from build123d import *
from build123d.topology import SkipClean

# Parameters (mm, degrees)
SKETCH1_R               = 10.5
SKETCH1_R_2             = 4
BOSS_EXTRUDE1_DEPTH     = 10
SKETCH1_3_R             = 4
BOSS_EXTRUDE2_DEPTH     = 17
CUT_EXTRUDE3_DEPTH      = 38.101212918
CUT_EXTRUDE3_DEPTH_BACK = 38.101212918
SKETCH4_R               = 5
HOLE1_D                 = 3
HOLE1_DEPTH             = 10
HOLE1_CBORE_D           = 4.5
HOLE1_CBORE_DEPTH       = 2
HOLE1_TIP               = 0.901290929
HOLE2_D                 = 11
HOLE2_DEPTH             = 7
SKETCH10_R              = 8.667878953
SKETCH10_R_2            = 2.5
CUT_EXTRUDE4_DEPTH      = 8


# Read off the part's stored shape, not the designer's step: M8x1.25 Machine Threads Stud1
with BuildPart() as part:
    # Sketch1 → Boss-Extrude1 (new body)
    # profile 1 of 2: a face of its own
    with BuildSketch(Plane(origin=(0, 0, 0), x_dir=(1, 0, 0), z_dir=(0, 1, 0))):
        with Locations(Location((0, 0, 0), (0, 0, 270))):
            Circle(SKETCH1_R)
        Circle(SKETCH1_R_2, mode=Mode.SUBTRACT)
    # profile 2 of 2: a face of its own
    with BuildSketch(Plane(origin=(0, 0, 0), x_dir=(1, 0, 0), z_dir=(0, 1, 0))):
        Circle(SKETCH1_R_2)
    extrude(amount=BOSS_EXTRUDE1_DEPTH)

    # Sketch1<3> → Boss-Extrude2 (add)
    with BuildSketch(Plane(origin=(0, 0, 0), x_dir=(1, 0, 0), z_dir=(0, 1, 0))):
        with Locations(Location((0, 0, 0), (0, 0, 270))):
            Circle(SKETCH1_3_R)
    extrude(amount=BOSS_EXTRUDE2_DEPTH)

    # M8x1.25 Machine Threads Stud1 outline → M8x1.25 Machine Threads Stud1 (revolve)
    with SkipClean():  # the faces are left unmerged after this step: merging them gives an invalid solid
        with BuildSketch(Plane.XY):
            Polygon((4, 17), (4, 33.3095), (3.3095, 34), (0, 34), (0, 17), align=None)
        revolve(axis=Axis((0, 0, 0), (0, 1, 0)))

    # Sketch4 → Cut-Extrude3 (cut, two sides: drawn at the far end of the back side and taken through both)
    with SkipClean():  # the faces are left unmerged after this step: merging them gives an invalid solid
        with BuildSketch(Plane(origin=(0, 0, 0), x_dir=(1, 0, 0), z_dir=(0, 1, 0)).offset(-CUT_EXTRUDE3_DEPTH_BACK)):
            with Locations((0, -13)):
                Circle(SKETCH4_R)
            with Locations((-11.258330249, 6.5)):
                Circle(SKETCH4_R)
            with Locations((11.258330249, 6.5)):
                Circle(SKETCH4_R)
        extrude(amount=CUT_EXTRUDE3_DEPTH + CUT_EXTRUDE3_DEPTH_BACK, mode=Mode.SUBTRACT)

    # Hole1
    with Locations(Plane(origin=(0, 10, 0), x_dir=(1, 0, 0), z_dir=(0, 1, 0))):
        with Locations((0, 7.505553499), (6.5, -3.75277675), (-6.5, -3.75277675)):
            CounterBoreHole(HOLE1_D / 2, HOLE1_CBORE_D / 2, HOLE1_CBORE_DEPTH, depth=HOLE1_DEPTH)
            with Locations((0, 0, -(HOLE1_DEPTH + HOLE1_TIP / 2))):  # 118° drill point
                Cone(0, HOLE1_D / 2, HOLE1_TIP, mode=Mode.SUBTRACT)

    # Hole2
    with Locations(Plane(origin=(0, 0, 0), x_dir=(-1, 0, 0), z_dir=(0, -1, 0))):
        with Locations((0, 0)):
            Hole(HOLE2_D / 2, depth=HOLE2_DEPTH)

    # Sketch10 → Cut-Extrude4 (cut)
    with SkipClean():  # the faces are left unmerged after this step: merging them gives an invalid solid
        with BuildSketch(Plane(origin=(0, 34, 0), x_dir=(1, 0, 0), z_dir=(0, 1, 0))):
            Circle(SKETCH10_R)
            with Locations(Location((0, 0, 0), (0, 0, 270))):
                Circle(SKETCH10_R_2, mode=Mode.SUBTRACT)
        extrude(amount=-CUT_EXTRUDE4_DEPTH, mode=Mode.SUBTRACT)
    add(part.part.scale(1), mode=Mode.REPLACE)  # the faces are merged on a copy


solid = part.part
Source: CAD feature listing. Evaluate the final solid. Frame: model axes, mm. A direction names the side the tool comes from. Coordinates: 2 decimals unless noted, no trailing zeros. Order: outer loops, then holes, each group sorted by start corner. A loop starts at its lowest first (then second) coordinate and runs counter-clockwise, first axis right, second up. Notation, with made-up numbers: M 36.5,50 L 94.5,50 A12 cw 94.5,61 Z; hole C 88.25,27.25 d6. An arc over 180 degrees is marked long. Write each question's results on one line, items separated by ' | '. Start each with the question number.
1. Pin query (flat end, axial travel): pin 1 (6 mm diameter, centred on x = 4.5, z = 3.5, fed in from +Y); pin 2 (5 mm diameter, centred on x = 5.5, y = 26.5, fed in from -Z); pin 3 (8 mm diameter, centred on x = 7.5, y = 23.5, fed in from +Z). Return the tip coordinate at first contact, or that it passes through.
2. Section B-B, the plane z = 0. Return the cut outline in (x, y), then the cut area to 3 significant figures.
3. Material intervals for L1, parallel to Z at x = 0, y = 5.75; L2, parallel to X at y = 2, z = 4.5; L3, parallel to Y at x = -2.75, z = 3, sorted ascending.
4. Section A-A, the plane x = 0. Return the cut outline in (y, z), then the cut area to 3 significant figures.
5. Reachability of faces 5 (the face through (2, 26, -2)), 6 (the face through (-5.394, 3.944, 2.739)), 7 (the face through (0, 7, 0)) from +Z, -Z, +X, -X, +Y, -Y: full face, straight path, thin tool, end or side. Return the list, or none.
6. Section D-D, the plane y = 12.5. Return the cut outline in (x, z).
7. Section C-C, the plane y = 27.5. Return the cut outline in (x, z).
8. Draft query along Z for faces 1 (the face through (0, 5, 8)), 2 (the face through (-1, 8, -6)), 3 (the face through (-0.293, 9.014, -9.736)), 4 (the face through (2, 10, 4)). Return one class per face: +Z half, -Z half, draft (parallel to the pull), parting line (faces both ways), or undercut.
Solution:
1) pin 1: y = 26 | pin 2: z = -2.59 | pin 3: z = 1.94
2) outline: M -10.5,0 L -5.5,0 L -5.5,7 L 5.5,7 L 5.5,0 L 10.5,0 L 10.5,10 L 4,10 L 4,26 L 2.5,26 L 2.5,34 L -2.5,34 L -2.5,26 L -4,26 L -4,10 L -10.5,10 Z | area: 301 mm²
3) L1: -10.5 to -9.01, -6.01 to -5.5, 5.5 to 8 | L2: -9.49 to -7.8, -5.2 to -3.16, 3.16 to 5.2, 7.8 to 9.49 | L3: 7 to 10
4) outline: M 0,-10.5 L 10,-10.5 L 10,-9.76 L 8,-9.76 L 8,-9.01 L 0,-9.01 Z; M 0,-6.01 L 8,-6.01 L 8,-5.26 L 10,-5.26 L 10,-4 L 26,-4 L 26,-2.5 L 34,-2.5 L 34,2.5 L 26,2.5 L 26,4 L 10,4 L 10,8 L 0,8 L 0,5.5 L 7,5.5 L 7,-5.5 L 0,-5.5 Z | area: 243 mm²
5) face 5: +Y | face 6: +Y, -Y | face 7: -Y
6) outline: C 0,0 d8
7) outline: C 0,0 d5
8) face 1: +Z half | face 2: undercut | face 3: undercut | face 4: draft
